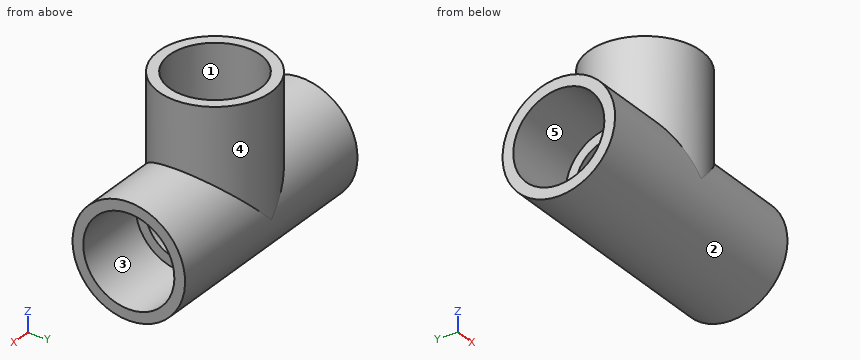
```python
from build123d import *

# Parameters (mm, degrees)
SOCKETRIGHT_R                       = 16.7005
SOCKETRIGHT_DEPTH                   = 29.68625
SOCKETRIGHT_PITCH_ANGLE             = 90
SOCKETTOP_R                         = 16.7005
SOCKETTOP_DEPTH                     = 29.68625
SOCKETLEFT_R                        = 16.7005
SOCKETLEFT_DEPTH                    = 29.68625
SOCKETLEFT_PITCH_ANGLE              = 90
OBJ1_R           = 13.0683
OBJ1_DEPTH       = 97.79
OBJ1_PITCH_ANGLE = 90
OBJ2             = 13.0683
OBJ3         = 48.895
OBJ4_R           = 20.6375
OBJ4_DEPTH       = 88.9
OBJ4_PITCH_ANGLE = 90
OBJ5             = 20.6375
OBJ6         = 44.45


with BuildPart() as socketright:
    # SocketRight → SocketRight (new body)
    with BuildSketch(Plane.XY):
        Circle(SOCKETRIGHT_R)
    extrude(amount=SOCKETRIGHT_DEPTH)


with BuildPart() as socketright_1:
    # SocketRight pitch: moved
    add(socketright.part.rotate(Axis((0, 0, 0), (0, 1, 0)), SOCKETRIGHT_PITCH_ANGLE))


with BuildPart() as socketright_2:
    # SocketRight placement: moved
    add(socketright_1.part.moved(Location((17.4625, 0, 0))))


with BuildPart() as sockettop:
    # SocketTop → SocketTop (new body)
    with BuildSketch(Plane.XY.offset(17.4625)):
        Circle(SOCKETTOP_R)
    extrude(amount=SOCKETTOP_DEPTH)


with BuildPart() as sockets:
    # SocketLeft → SocketLeft (new body)
    with BuildSketch(Plane.XY):
        Circle(SOCKETLEFT_R)
    extrude(amount=SOCKETLEFT_DEPTH)


with BuildPart() as sockets_1:
    # SocketLeft pitch: moved
    add(sockets.part.rotate(Axis((0, 0, 0), (0, 1, 0)), SOCKETLEFT_PITCH_ANGLE))


with BuildPart() as sockets_2:
    # SocketLeft placement: moved
    add(sockets_1.part.moved(Location((-47.14875, 0, 0))))

    # Sockets: union SocketRight, SocketTop
    add(socketright_2.part)
    add(sockettop.part)


with BuildPart() as obj1:
    # obj1 → obj1 (new body)
    with BuildSketch(Plane.XY):
        Circle(OBJ1_R)
    extrude(amount=OBJ1_DEPTH)


with BuildPart() as obj1_1:
    # obj1 pitch: moved
    add(obj1.part.rotate(Axis((0, 0, 0), (0, 1, 0)), OBJ1_PITCH_ANGLE))


with BuildPart() as obj1_2:
    # obj1 placement: moved
    add(obj1_1.part.moved(Location((-48.895, 0, 0))))


with BuildPart() as innerteefusion:
    with BuildSketch(Plane.XY):
        Circle(OBJ2)
    extrude(amount=OBJ3)

    # InnerTeeFusion: union obj1
    add(obj1_2.part)


with BuildPart() as obj4:
    # obj4 → obj4 (new body)
    with BuildSketch(Plane.XY):
        Circle(OBJ4_R)
    extrude(amount=OBJ4_DEPTH)


with BuildPart() as obj4_1:
    # obj4 pitch: moved
    add(obj4.part.rotate(Axis((0, 0, 0), (0, 1, 0)), OBJ4_PITCH_ANGLE))


with BuildPart() as obj4_2:
    # obj4 placement: moved
    add(obj4_1.part.moved(Location((-44.45, 0, 0))))


with BuildPart() as tee:
    with BuildSketch(Plane.XY):
        Circle(OBJ5)
    extrude(amount=OBJ6)

    # OuterTeeFusion: union obj4
    add(obj4_2.part)

    # Cut: cut InnerTeeFusion
    add(innerteefusion.part, mode=Mode.SUBTRACT)

    # Tee: cut Sockets
    add(sockets_2.part, mode=Mode.SUBTRACT)


solid = tee.part
```
Input: part model. Units: mm. Frame: model coordinates. Face numbers are marked on the shaded views. A direction names the side the tool comes from. Coordinates: 2 decimals unless noted, no trailing zeros. Write each loop counter-clockwise with the first axis right and the second up, starting at its lowest first coordinate (ties: lowest second). Pieces come first, ordered by that corner, then holes. Notation, with made-up numbers: M 28,59.25 L 73,59.25 A22 ccw 73,95.25 Z; hole C 78,47.25 d4. An arc over 180 degrees is marked long. Use one line per item in the form item = value.
Q1. Draft query along Z for the marked faces 1, 2 and 3. Return one class per face: released by +Z, released by -Z, zero draft, split by the parting line, or undercut.
Answer below:
face_1 = zero draft
face_2 = split by the parting line
face_3 = undercut
Q2. Section A-A (y = 0). Return loops of the section in (x, z), plus the area to 3 significant figures.
Answer below:
outline = M -44.45,-20.64 L 44.45,-20.64 L 44.45,-16.7 L 17.46,-16.7 L 17.46,-13.07 L -17.46,-13.07 L -17.46,-16.7 L -44.45,-16.7 Z; M -44.45,16.7 L -17.46,16.7 L -17.46,13.07 L -13.07,13.07 L -13.07,17.46 L -16.7,17.46 L -16.7,44.45 L -20.64,44.45 L -20.64,20.64 L -44.45,20.64 Z; M 13.07,13.07 L 17.46,13.07 L 17.46,16.7 L 44.45,16.7 L 44.45,20.64 L 20.64,20.64 L 20.64,44.45 L 16.7,44.45 L 16.7,17.46 L 13.07,17.46 Z
area = 920 mm²
Q3. First-contact query: pin 1 (6 mm diameter, centred on y = -13.5, z = 7, fed in from -X); pin 2 (4 mm diameter, centred on y = -5, z = 28.5, fed in from -X); pin 3 (6 mm diameter, centred on y = -11, z = 6.5, fed in from -X); pin 4 (3 mm diameter, centred on x = 18, z = -9.5, fed in from +Y). Flat tips, straight axial feed; report the tip coordinate or a pass-through.
Answer below:
pin_1 = -44.45
pin_2 = -20.42
pin_3 = -17.46
pin_4 = 19.02
Q4. Material intervals for probe 1 along Y at (x, z) = (-28, 0), sorted ascending. Write a range as from..to.
Answer below:
probe_1 = -20.64..-16.7, 16.7..20.64
Q5. Set-up query: the marked faces 4 and 5. Return all of +Z, -Z, +X, -X, +Y, -Y with unobstructed straight access to the full face (end or side cutting, diameter ignored); none if empty.
Answer below:
face_4 = +Z
face_5 = -X
